Part model, mm, in its own coordinate system. A direction names the side the tool comes from. Coordinates: 2 decimals unless noted, no trailing zeros. Order: outer loops, then holes, each group sorted by start corner. A loop starts at its lowest first (then second) coordinate and runs counter-clockwise, first axis right, second up.
from build123d import *

# Parameters (mm, degrees)
SKETCH1_R           = 1.5
BOSS_EXTRUDE1_DEPTH = 3.175
SKETCH2_R           = 4
BOSS_EXTRUDE2_DEPTH = 10
FILLET1_R           = 1
SKETCH3_R           = 1.1
CUT_EXTRUDE1_DEPTH  = 5


with BuildPart() as part:
    # Sketch1 → Boss-Extrude1 (new body)
    with BuildSketch(Plane(origin=(0, 0, 0), x_dir=(1, 0, 0), z_dir=(0, 1, 0))):
        with BuildLine():
            Line((3.570714214, 3.5), (27.570714214, 3.5))
            Line((27.570714214, 3.5), (27.570714214, -3.5))
            Line((27.570714214, -3.5), (3.570714214, -3.5))
            ThreePointArc((3.570714214, -3.5), (-5, 0), (3.570714214, 3.5))
        make_face()
        with Locations(Location((8.9, 0, 0), (0, 0, 270))):
            Circle(SKETCH1_R, mode=Mode.SUBTRACT)
        with Locations(Location((20, 0, 0), (0, 0, 270))):
            Circle(SKETCH1_R, mode=Mode.SUBTRACT)
        with Locations(Location((24, 0, 0), (0, 0, 270))):
            Circle(SKETCH1_R, mode=Mode.SUBTRACT)
    extrude(amount=BOSS_EXTRUDE1_DEPTH)

    # Sketch2 → Boss-Extrude2 (add)
    with BuildSketch(Plane(origin=(0, 3.175, 0), x_dir=(1, 0, 0), z_dir=(0, 1, 0))):
        with Locations(Location((0, 0, 0), (0, 0, 270))):
            Circle(SKETCH2_R)
    extrude(amount=BOSS_EXTRUDE2_DEPTH)

    # Fillet1
    fillet1_edges = [part.edges().sort_by_distance(p)[0] for p in [
        (27.570714214, 1.5875, 3.5),
        (3.570714214, 1.5875, 3.5),
        (3.570714214, 1.5875, -3.5),
        (27.570714214, 1.5875, -3.5),
    ]]
    fillet(fillet1_edges, radius=FILLET1_R)

    # Sketch3 → Cut-Extrude1 (cut)
    with BuildSketch(Plane(origin=(0, 13.175, 0), x_dir=(1, 0, 0), z_dir=(0, 1, 0))):
        with Locations(Location((2, 0, 0), (0, 0, 270))):
            Circle(SKETCH3_R)
        with Locations(Location((-2, 0, 0), (0, 0, 270))):
            Circle(SKETCH3_R)
    extrude(amount=-CUT_EXTRUDE1_DEPTH, mode=Mode.SUBTRACT)


solid = part.part
Q1. Pin check, flat tips, straight feed: pin 1 Ø5 at (x, z) = (20, 0) entering from -Y; pin 2 Ø1.5 at (x, z) = (13.5, 0.5) entering from +Y (3 decimals); pin 3 Ø2 at (y, z) = (11, 3) entering from -X; pin 4 Ø0.7 at (x, z) = (-1.5, 0) entering from +Y (3 decimals). Stop position of each tip, or through.
Results list:
pin 1: stops at y = 0
pin 2: stops at y = 3.175
pin 3: stops at x = -3.46
pin 4: stops at y = 8.175
Q2. Cut at D-D on x = 0. Write the cut outline in (y, z) (3 decimals).
Results list:
outline: (0, -5) - (3.175, -5) - (3.175, -4) - (13.175, -4) - (13.175, 4) - (3.175, 4) - (3.175, 5) - (0, 5) - close
Q3. Which spindle directions (+Z, -Z, +X, -X, +Y, -Y) get a long thin tool onto all of the face, cutting with end or side? Do faces 1 (the face through (-5, 2, 0)), 2 (the face through (-3.905, 8.105, -0.867)), 3 (the face through (15, 2, -3.5)). Say none if no direction does.
Results list:
face 1: +Y, -Y
face 2: +Y
face 3: -Z, +X, +Y, -Y
Q4. Cut at A-A on z = 0. Write the cut outline in (x, y) (3 decimals).
Results list:
outline: (-5, 0) - (7.4, 0) - (7.4, 3.175) - (4, 3.175) - (4, 13.175) - (3.1, 13.175) - (3.1, 8.175) - (0.9, 8.175) - (0.9, 13.175) - (-0.9, 13.175) - (-0.9, 8.175) - (-3.1, 8.175) - (-3.1, 13.175) - (-4, 13.175) - (-4, 3.175) - (-5, 3.175) - close; (10.4, 0) - (18.5, 0) - (18.5, 3.175) - (10.4, 3.175) - close; (21.5, 0) - (22.5, 0) - (22.5, 3.175) - (21.5, 3.175) - close; (25.5, 0) - (27.571, 0) - (27.571, 3.175) - (25.5, 3.175) - close
Q5. Mould opens along Z. For faces 4 (the face through (0.926, 10.71, -0.238)), 5 (the face through (15, 2, 3.5)), 6 (the face through (0, 13.175, 0)) say: pulls with the +Z half, pulls with the -Z half, needs draft (parallel to the pull), parting line crosses it, or undercut.
Results list:
face 4: undercut
face 5: pulls with the +Z half
face 6: needs draft
Q6. Cut at C-C on y = 2. Write the cut outline in (x, z).
Results list:
outline: (3.31, -3.75) arc R1 cw to (3.97, -3.5) - (26.57, -3.5) arc R1 ccw to (27.57, -2.5) - (27.57, 2.5) arc R1 ccw to (26.57, 3.5) - (3.97, 3.5) arc R1 cw to (3.31, 3.75) arc R5 ccw (long way) to start; hole circle Ø3 at (8.9, 0); hole circle Ø3 at (20, 0); hole circle Ø3 at (24, 0)
Q7. Wall check: line 1 along X through (y, z) = (1.9, 0); line 2 along X through (y, z) = (10.75, 1); line 3 along X through (y, z) = (11, -0.5). Give the ranges that are in metal, low to high.
Results list:
line 1: x = -5 to 7.4, 10.4 to 18.5, 21.5 to 22.5, 25.5 to 27.57
line 2: x = -3.87 to -2.46, -1.54 to 1.54, 2.46 to 3.87
line 3: x = -3.97 to -2.98, -1.02 to 1.02, 2.98 to 3.97
Q8. Cut at B-B on x = 24. Write the cut outline in (y, z) (3 decimals).
Results list:
outline: (0, -3.5) - (3.175, -3.5) - (3.175, -1.5) - (0, -1.5) - close; (0, 1.5) - (3.175, 1.5) - (3.175, 3.5) - (0, 3.5) - close
